Design review of the part built by this model. Coordinates are the model's own, in mm. Round coordinates to 2 decimals unless told otherwise and drop trailing zeros. Order: outer loops, then holes, each group sorted by start corner. A loop starts at its lowest first (then second) coordinate and runs counter-clockwise, first axis right, second up. Notation, with made-up numbers: (-9, 36) - (7, 36) arc R21 cw to (7, 45) - close; hole circle Ø6 at (10, -38.75). An arc over 180 degrees is marked (long way). Write item = value, one per line.
from build123d import *

# Parameters (mm, degrees)
BOSS_EXTRUDE1_DEPTH = 4
SKETCH3_R           = 8
BOSS_EXTRUDE2_DEPTH = 4
SKETCH3_2_R         = 8
CUT_EXTRUDE1_DEPTH  = 4


with BuildPart() as part:
    # Sketch1 → Boss-Extrude1 (new body)
    with BuildSketch(Plane.XY):
        Polygon((-20, 140), (-20, -140), (-20, -200), (20, -200), (20, -140), (20, 140), (20, 200), (-20, 200), align=None)
    extrude(amount=BOSS_EXTRUDE1_DEPTH)

    # Sketch3 → Boss-Extrude2 (add)
    with BuildSketch(Plane(origin=(0, 0, 0), x_dir=(-1, 0, 0), z_dir=(0, 0, -1))):
        with Locations((0, 90)):
            Circle(SKETCH3_R)
        with Locations((0, -50)):
            Circle(SKETCH3_R)
    extrude(amount=-BOSS_EXTRUDE2_DEPTH)

    # Sketch3<2> → Cut-Extrude1 (cut)
    with BuildSketch(Plane(origin=(0, 0, 0), x_dir=(-1, 0, 0), z_dir=(0, 0, -1))):
        with Locations((0, 90)):
            Circle(SKETCH3_2_R)
        with Locations((0, -50)):
            Circle(SKETCH3_2_R)
    extrude(amount=-CUT_EXTRUDE1_DEPTH, mode=Mode.SUBTRACT)


solid = part.part
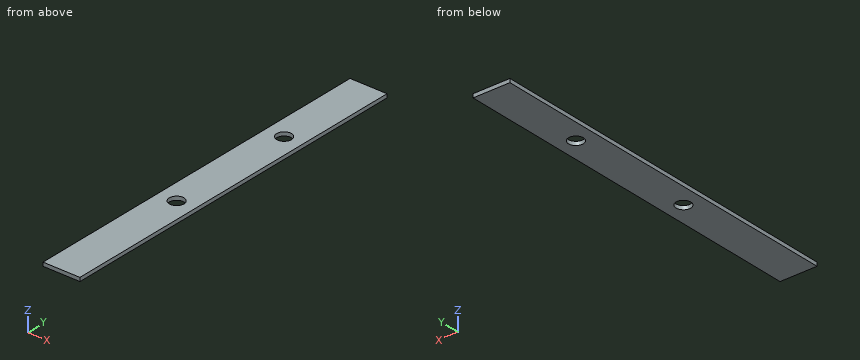
Item 1: For line 1 along Y through (x, z) = (0, 0.95); line 2 along X through (y, z) = (89, 2.3); line 3 along Y through (x, z) = (-5.5, 2.4), list the stretches that pass through material, from the lowest coordinate up. Write a range as [from, to].
Data:
line_1 = [-200, -58], [-42, 82], [98, 200]
line_2 = [-20, -7.94], [7.94, 20]
line_3 = [-200, -55.81], [-44.19, 84.19], [95.81, 200]
Item 2: Insertion check: P1, Ø13, axis at x = 0, y = 90, coming from the -Z side. The pin has a flat end and moves straight along its axis. Give the tip position at first contact, or say it passes through.
Data:
P1 = through
Item 3: Take a section at C-C, the plane z = 0.9. State the section outline as (x, y) points.
Data:
outline = (-20, -200) - (20, -200) - (20, 200) - (-20, 200) - close; hole circle Ø16 at (0, -50); hole circle Ø16 at (0, 90)
Item 4: Take a section at B-B, the plane y = -50. State the section outline as (x, z) points, and give its area (3 significant figures).
Data:
outline = (-20, 0) - (-8, 0) - (-8, 4) - (-20, 4) - close; (8, 0) - (20, 0) - (20, 4) - (8, 4) - close
area = 96.0 mm2
Item 5: Take a section at A-A, the plane x = 0. State the section outline as (y, z) points.
Data:
outline = (-200, 0) - (-58, 0) - (-58, 4) - (-200, 4) - close; (-42, 0) - (82, 0) - (82, 4) - (-42, 4) - close; (98, 0) - (200, 0) - (200, 4) - (98, 4) - close
